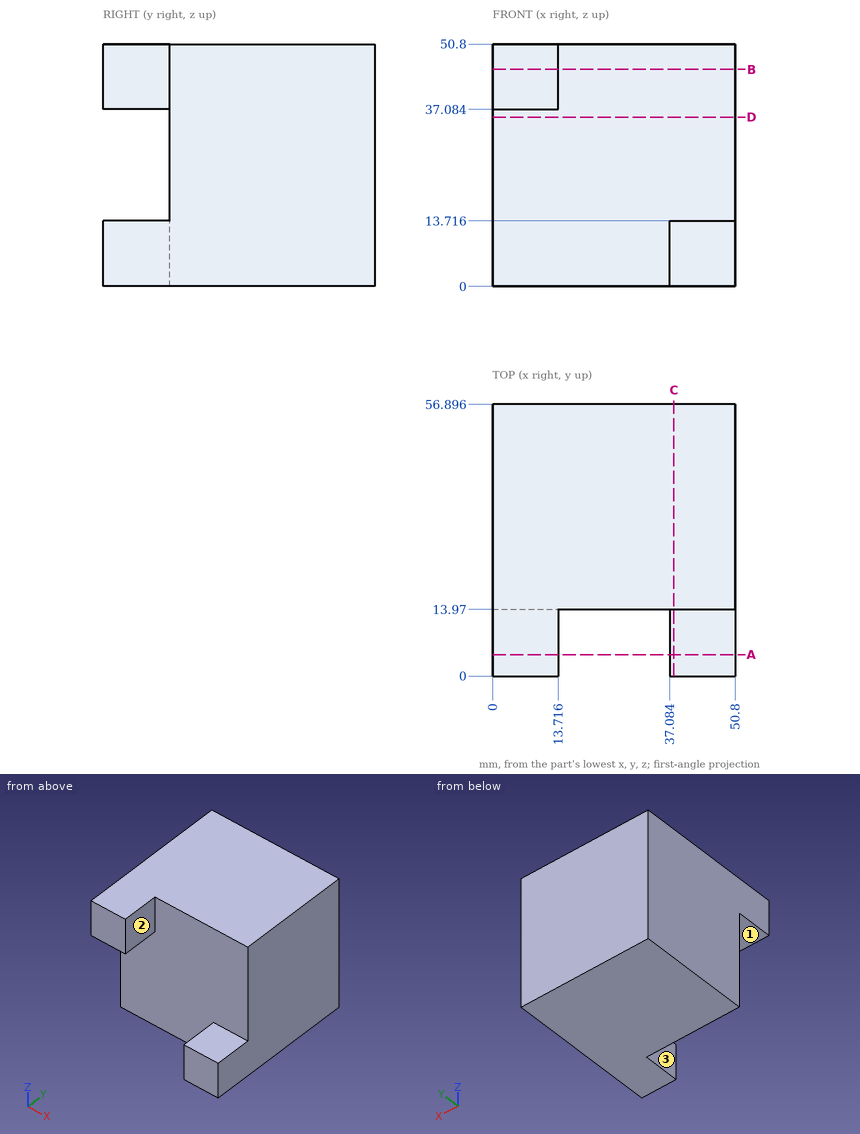
Design review of the part shown in the three views and the two pictorial views. Dimensions are in mm from the part's minimum x, y and z. A direction names the side the tool comes from. Coordinates: 2 decimals unless noted, no trailing zeros. Write each loop counter-clockwise with the first axis right and the second up, starting at its lowest first coordinate (ties: lowest second). Pieces come first, ordered by that corner, then holes.
(1) Tool access review of the marked faces 1, 2 and 3: name each direction out of +Z, -Z, +X, -X, +Y, -Y from which nothing blocks a thin tool from reaching the whole face with its end or side.
(2) Add section A-A on y = 4.5. Give the boundary of the cut face in (x, z), then the cut area to 3 significant figures.
(3) For pin 1 Ø7 at (y, z) = (6.5, 5) entering from -X; pin 2 Ø1 at (x, z) = (14.5, 31.5) entering from -Y; pin 3 Ø4 at (x, y) = (7.5, 8.5) entering from -Z, all flat-tipped, find the tip position at first contact; note any pin that passes through.
(4) Wall thickness on probe 1 along Y at (x, z) = (46, 15.5); probe 2 along Z at (x, y) = (2, 11.5); probe 3 along X at (y, z) = (13, 45.5): over which ranges is each line inside the solid? List them lowest first.
(5) Add section B-B on z = 45.5. Give the boundary of the cut face in (x, y).
(6) Add section D-D on z = 35.5. Give the boundary of the cut face in (x, y), then the cut area to 3 significant figures.
(7) Add section C-C on x = 38. Give the boundary of the cut face in (y, z).
Answer sheet:
1. face 1: -Z, +X, -X, -Y
1. face 2: +Z, -Z, +X, -Y
1. face 3: +Z, -Z, -X, -Y
2. outline: (0, 37.08) - (13.72, 37.08) - (13.72, 50.8) - (0, 50.8) - close; (37.08, 0) - (50.8, 0) - (50.8, 13.72) - (37.08, 13.72) - close
2. area: 376 mm2
3. pin 1: stops at x = 37.08
3. pin 2: stops at y = 13.97
3. pin 3: stops at z = 37.08
4. probe 1: y = 13.97 to 56.9
4. probe 2: z = 37.08 to 50.8
4. probe 3: x = 0 to 13.72
5. outline: (0, 0) - (13.72, 0) - (13.72, 13.97) - (50.8, 13.97) - (50.8, 56.9) - (0, 56.9) - close
6. outline: (0, 13.97) - (50.8, 13.97) - (50.8, 56.9) - (0, 56.9) - close
6. area: 2,180 mm2
7. outline: (0, 0) - (56.9, 0) - (56.9, 50.8) - (13.97, 50.8) - (13.97, 13.72) - (0, 13.72) - close
